Work out the finished part from the listing and answer in its coordinate system (mm). Face numbers are marked on the shaded views. A direction names the side the tool comes from. Give positions to 0.01 mm unless a question says otherwise; leave off trailing zeros. Order: outer loops, then holes, each group sorted by start corner. A loop starts at its lowest first (then second) coordinate and runs counter-clockwise, first axis right, second up.
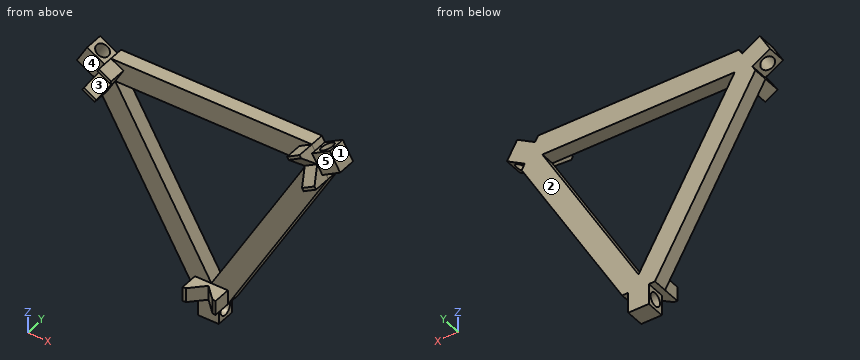
```python
from build123d import *

# Parameters (mm, degrees)
BOSS_EXTRUDE1_DEPTH          = 1.778
BOSS_EXTRUDE2_DEPTH          = 2.159
CUT_EXTRUDE1_DEPTH           = 28.428162383
BOSS_EXTRUDE4_DEPTH          = 2.286
F_97_0_0059_DIAMETER_HOLE1_D = 1.651
CIRPATTERN2_COUNT            = 3
CIRPATTERN3_COUNT            = 3


with BuildPart() as part:
    # Sketch1 → Boss-Extrude1 (new body)
    with BuildSketch(Plane(origin=(0, 0, 0), x_dir=(1, 0, 0), z_dir=(0, 1, 0))):
        Polygon((-2.032, 15.494), (-14.434197606, -5.98723638), (-13.418197606, -7.747), (-12.402197606, -9.50676362), (12.402197606, -9.50676362), (13.418197606, -7.747), (14.434197606, -5.98723638), (2.032, 15.494), (0, 15.494), align=None)
        Polygon((0, 13.716), (-11.878404438, -6.858), (11.878404438, -6.858), align=None, mode=Mode.SUBTRACT)
    extrude(amount=BOSS_EXTRUDE1_DEPTH)

    # Sketch3 → Boss-Extrude2 (add)
    with BuildSketch(Plane(origin=(0, 0, 0), x_dir=(-1, 0, 0), z_dir=(0, -1, 0))):
        Polygon((0, 13.716), (2.032, 13.716), (2.032, 15.494), (-2.032, 15.494), (-2.032, 13.716), align=None)
    boss_extrude2 = extrude(amount=BOSS_EXTRUDE2_DEPTH)

    # Sketch4 → Cut-Extrude1 (cut, through all)
    with BuildSketch(Plane.XY.offset(-13.716)):
        Polygon((0, -0.508), (-2.694076836, -3.202076836), (2.694076836, -3.202076836), align=None)
    cut_extrude1 = extrude(amount=-CUT_EXTRUDE1_DEPTH, mode=Mode.SUBTRACT)

    # Sketch6 → Boss-Extrude4 (add)
    with BuildSketch(Plane(origin=(0, 1.778, 0), x_dir=(1, 0, 0), z_dir=(0, 1, 0))):
        Polygon((0, 15.494), (1.27, 15.494), (1.27, 18.034), (-1.27, 18.034), (-1.27, 15.494), align=None)
    boss_extrude4 = extrude(amount=-BOSS_EXTRUDE4_DEPTH)

    # #97 (0.0059) Diameter Hole1 (through all)
    with Locations(Plane(origin=(1.27, 0, 0), x_dir=(0, 0, -1), z_dir=(1, 0, 0))):
        with Locations((16.764, 0.635)):
            f_97_0_0059_diameter_hole1 = Hole(F_97_0_0059_DIAMETER_HOLE1_D / 2)

    # CirPattern2: Boss-Extrude2, Cut-Extrude1 ×3 about axis
    cirpattern2_axis = Axis((0, 0, 0), (0, 1, 0))
    add([boss_extrude2.rotate(cirpattern2_axis, i * 360 / CIRPATTERN2_COUNT) for i in range(1, CIRPATTERN2_COUNT)])
    add([cut_extrude1.rotate(cirpattern2_axis, i * 360 / CIRPATTERN2_COUNT) for i in range(1, CIRPATTERN2_COUNT)], mode=Mode.SUBTRACT)

    # CirPattern3: Boss-Extrude4, #97 (0.0059) Diameter Hole1 ×3 about axis
    cirpattern3_axis = Axis((0, 0, 0), (0, 1, 0))
    add([boss_extrude4.rotate(cirpattern3_axis, i * 360 / CIRPATTERN3_COUNT) for i in range(1, CIRPATTERN3_COUNT)])
    add([f_97_0_0059_diameter_hole1.rotate(cirpattern3_axis, i * 360 / CIRPATTERN3_COUNT) for i in range(1, CIRPATTERN3_COUNT)], mode=Mode.SUBTRACT)


solid = part.part
```
1. The mould has two halves that part along X. Classify the marked faces 1, 2 and 3: pulls with the +X half, pulls with the -X half, needs draft (parallel to the pull), parting line crosses it, or undercut.
Findings below:
face 1: pulls with the +X half
face 2: needs draft
face 3: undercut
2. Straight lines are drawn through the part: probe 1 along X at (y, z) = (-0.95, -14.5); probe 2 along Z at (x, y) = (-8, 0.5); probe 3 along Z at (x, y) = (-3.5, 0.55). For each, find the intervals that lie inside material, in ascending order.
Findings below:
probe 1: x = -2.03 to -0.44, 0.44 to 2.03
probe 2: z = -5.16 to 0.14, 6.86 to 9.51
probe 3: z = -12.95 to -7.65, 6.86 to 9.51
3. Given P1, Ø5, axis at x = -3, z = -4.5, coming from the +Y side; P2, Ø1.4, axis at y = -1.5, z = -14.5, coming from the +X side; P3, Ø0.9, axis at x = 3, y = 0.5, coming from the -Z side; P4, Ø1.1, axis at x = -1, y = -1, coming from the +Z side, each flat-ended and moving along its own axis, determine where each tip first touches the part or whether it passes through.
Findings below:
P1: stops at y = 1.78
P2: stops at x = 2.03
P3: stops at z = -14.6
P4: stops at z = -13.72
4. Which of the six approach directions +Z, -Z, +X, -X, +Y, -Y give full straight-line access (tool end or side, diameter ignored) to the marked faces 4 and 5?
Findings below:
face 4: +Z, -X, -Y
face 5: +Z, +X, -Y
5. The part is cut by section B-B (x = -11.5). Write down the section's boundary in (y, z).
Findings below:
outline: (-2.16, 8.55) - (-1.26, 7.51) - (0, 7.51) - (0, 6.86) - (1.78, 6.86) - (1.78, 9.51) - (0, 9.51) - (0, 8.99) - (-2.16, 8.99) - close; (0, 0.91) - (1.78, 0.91) - (1.78, 6.2) - (0, 6.2) - close
6. The part is cut by section A-A (z = -0.25). Write down the section's boundary in (x, y).
Findings below:
outline: (-10.83, 0) - (-7.77, 0) - (-7.77, 1.78) - (-10.83, 1.78) - close; (7.77, 0) - (10.83, 0) - (10.83, 1.78) - (7.77, 1.78) - close
7. The part is cut by section C-C (y = -1.1). Write down the section's boundary in (x, z), then the cut area to 3 significant figures.
Findings below:
outline: (-14.43, 5.99) - (-12.89, 5.1) - (-12.17, 6.35) - (-13.71, 7.23) - close; (-13.12, 8.26) - (-11.58, 7.37) - (-10.86, 8.62) - (-12.4, 9.51) - close; (-2.03, -15.49) - (-0.59, -15.49) - (-0.59, -13.72) - (-2.03, -13.72) - close; (0.59, -15.49) - (2.03, -15.49) - (2.03, -13.72) - (0.59, -13.72) - close; (10.86, 8.62) - (11.58, 7.37) - (13.12, 8.26) - (12.4, 9.51) - close; (12.17, 6.35) - (12.89, 5.1) - (14.43, 5.99) - (13.71, 7.23) - close
area: 15.4 mm2
8. The part is cut by section D-D (x = -5). Write down the section's boundary in (y, z).
Findings below:
outline: (0, -10.35) - (1.78, -10.35) - (1.78, -5.06) - (0, -5.06) - close; (0, 6.86) - (1.78, 6.86) - (1.78, 9.51) - (0, 9.51) - close
